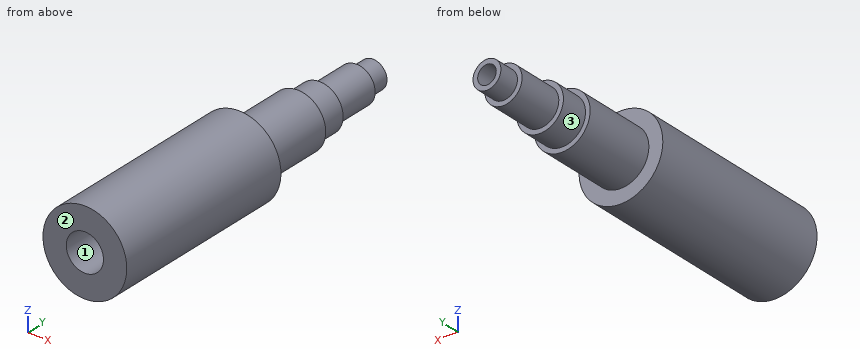
from build123d import *

# Parameters (mm, degrees)
SKETCH1_R                 = 9
BASE_SECTION_DEPTH        = 42
SKETCH2_R                 = 6
SECOND_SECTION_DEPTH      = 16
SKETCH3_R                 = 5
BEARING_SECTION_DEPTH     = 6
SKETCH4_R                 = 4
SEAL_SECTION_DEPTH        = 10
SKETCH5_R                 = 3
IMPELLER_SECTION_DEPTH    = 4.5
SKETCH6_R                 = 2
IMPELLER_SCREW_HOLE_DEPTH = 10
SKETCH7_R                 = 4
MOTOR_SHAFT_HOLE_DEPTH    = 32


with BuildPart() as part:
    # Sketch1 → base section (new body)
    with BuildSketch(Plane(origin=(0, 0, 0), x_dir=(1, 0, 0), z_dir=(0, 1, 0))):
        with Locations(Location((0, 0, 0), (0, 0, 90))):
            Circle(SKETCH1_R)
    extrude(amount=BASE_SECTION_DEPTH)

    # Sketch2 → second section (add)
    with BuildSketch(Plane(origin=(0, 42, 0), x_dir=(1, 0, 0), z_dir=(0, 1, 0))):
        with Locations(Location((0, 0, 0), (0, 0, 270))):
            Circle(SKETCH2_R)
    extrude(amount=SECOND_SECTION_DEPTH)

    # Sketch3 → bearing section (add)
    with BuildSketch(Plane(origin=(0, 58, 0), x_dir=(1, 0, 0), z_dir=(0, 1, 0))):
        with Locations(Location((0, 0, 0), (0, 0, 270))):
            Circle(SKETCH3_R)
    extrude(amount=BEARING_SECTION_DEPTH)

    # Sketch4 → seal section (add)
    with BuildSketch(Plane(origin=(0, 64, 0), x_dir=(1, 0, 0), z_dir=(0, 1, 0))):
        with Locations(Location((0, 0, 0), (0, 0, 270))):
            Circle(SKETCH4_R)
    extrude(amount=SEAL_SECTION_DEPTH)

    # Sketch5 → impeller section (add)
    with BuildSketch(Plane(origin=(0, 74, 0), x_dir=(1, 0, 0), z_dir=(0, 1, 0))):
        with Locations(Location((0, 0, 0), (0, 0, 270))):
            Circle(SKETCH5_R)
    extrude(amount=IMPELLER_SECTION_DEPTH)

    # Sketch6 → impeller screw hole (cut)
    with BuildSketch(Plane(origin=(0, 78.5, 0), x_dir=(1, 0, 0), z_dir=(0, 1, 0))):
        with Locations(Location((0, 0, 0), (0, 0, 270))):
            Circle(SKETCH6_R)
    extrude(amount=-IMPELLER_SCREW_HOLE_DEPTH, mode=Mode.SUBTRACT)

    # Sketch7 → motor shaft hole (cut)
    with BuildSketch(Plane(origin=(0, 0, 0), x_dir=(-1, 0, 0), z_dir=(0, -1, 0))):
        with Locations(Location((0, 0, 0), (0, 0, 270))):
            Circle(SKETCH7_R)
    extrude(amount=-MOTOR_SHAFT_HOLE_DEPTH, mode=Mode.SUBTRACT)


solid = part.part
Check sheet for the modelled part. Datum: model origin and axes. Units: mm. Face numbers are marked on the shaded views. A direction names the side the tool comes from. Coordinates: 2 decimals unless noted, no trailing zeros. Loops run counter-clockwise (first coordinate to the right, second up) from the corner with the lowest first, then second, coordinate; pieces in that order, holes last. Notation, with made-up numbers: (-12, -9.5) -> (3, -9.5) arc R33 ccw to (3, 23.5) -> close; hole circle Ø6 at (-19.75, -27). An arc over 180 degrees is marked (long way). Write item = value, one per line. Start each with the question number.
1. Tool access check on the marked faces 1, 2 and 3. Record the directions out of +Z, -Z, +X, -X, +Y, -Y that give a thin tool (end or side, any length) a straight path to the whole face; none if there is none.
2. Depth check by flat-ended pin: P1, Ø3.5, axis at x = 0, z = 0, coming from the -Y side; P2, Ø6, axis at x = -6.5, y = 24.5, coming from the +Z side; P3, Ø5, axis at x = -3, y = 59.5, coming from the -Z side. Enter the tip coordinate at first touch or a pass-through.
3. Material ranges on line 1 (X direction, y = 12, z = 0); line 2 (X direction, y = 73.75, z = 0); line 3 (Y direction, x = 4.75, z = -7), recorded low to high.
4. Section check C-C on x = 0. Record the cut outline in (y, z).
5. Section check B-B on y = 5.5. Record the cut outline in (x, z).
6. Section check D-D on z = -7.25. Record the cut outline in (x, y), then the cut area to 3 significant figures.
7. Section check A-A on z = 0. Record the cut outline in (x, y), then the cut area to 3 significant figures.
Responses:
q1.face_1 = -Y
q1.face_2 = +Z, -Z, +X, -X, -Y
q1.face_3 = +Y
q2.P1 = 32
q2.P2 = 8.29
q2.P3 = -5.92
q3.line_1 = -9 to -4, 4 to 9
q3.line_2 = -4 to -2, 2 to 4
q3.line_3 = 0 to 42
q4.outline = (0, -9) -> (42, -9) -> (42, -6) -> (58, -6) -> (58, -5) -> (64, -5) -> (64, -4) -> (74, -4) -> (74, -3) -> (78.5, -3) -> (78.5, -2) -> (68.5, -2) -> (68.5, 2) -> (78.5, 2) -> (78.5, 3) -> (74, 3) -> (74, 4) -> (64, 4) -> (64, 5) -> (58, 5) -> (58, 6) -> (42, 6) -> (42, 9) -> (0, 9) -> (0, 4) -> (32, 4) -> (32, -4) -> (0, -4) -> close
q5.outline = circle Ø18 at (0, 0); hole circle Ø8 at (0, 0)
q6.outline = (-5.33, 0) -> (5.33, 0) -> (5.33, 42) -> (-5.33, 42) -> close
q6.area = 448 mm2
q7.outline = (-9, 0) -> (-4, 0) -> (-4, 32) -> (4, 32) -> (4, 0) -> (9, 0) -> (9, 42) -> (6, 42) -> (6, 58) -> (5, 58) -> (5, 64) -> (4, 64) -> (4, 74) -> (3, 74) -> (3, 78.5) -> (2, 78.5) -> (2, 68.5) -> (-2, 68.5) -> (-2, 78.5) -> (-3, 78.5) -> (-3, 74) -> (-4, 74) -> (-4, 64) -> (-5, 64) -> (-5, 58) -> (-6, 58) -> (-6, 42) -> (-9, 42) -> close
q7.area = 819 mm2
